Geometry check sheet. Reference: the model listing, model coordinates, mm. Face numbers are marked on the shaded views. A direction names the side the tool comes from. Coordinates: 2 decimals unless noted, no trailing zeros. Order: outer loops, then holes, each group sorted by start corner. A loop starts at its lowest first (then second) coordinate and runs counter-clockwise, first axis right, second up.
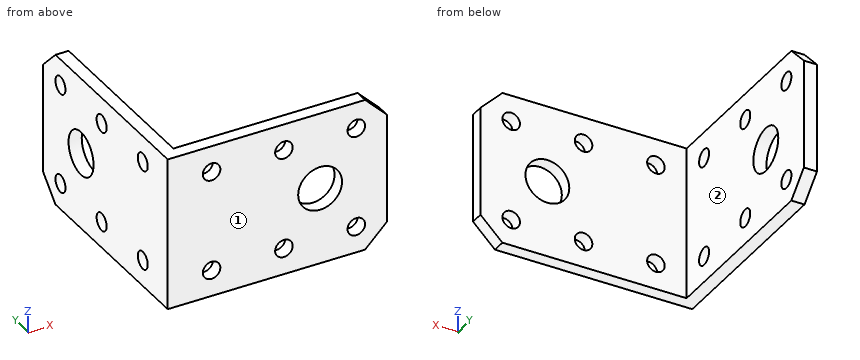
```python
from build123d import *

# Parameters (mm, degrees)
F1_DEPTH = 35
F2_R     = 5
F2_R_2   = 2
F3_DEPTH = 3
F4_R     = 5
F4_R_2   = 2
F5_DEPTH = 3
F6_SIZE  = 5
F7_SIZE  = 5


with BuildPart() as f1:
    # F0 (on Top) → F1 (new body)
    with BuildSketch(Plane.XY):
        Polygon((0, 50), (0, 0), (50, 0), (50, 3), (3, 3), (3, 50), align=None)
    extrude(amount=F1_DEPTH)

    # F2 (on face) → F3 (cut, through all)
    with BuildSketch(Plane(origin=(0, 3, 0), x_dir=(-1, 0, 0), z_dir=(0, 1, 0))):
        with Locations((-34.75, 17.5)):
            Circle(F2_R)
        with Locations((-43, 29)):
            Circle(F2_R_2)
        with Locations((-26.5, 29)):
            Circle(F2_R_2)
        with Locations((-10, 29)):
            Circle(F2_R_2)
        with Locations((-43, 6)):
            Circle(F2_R_2)
        with Locations((-26.5, 6)):
            Circle(F2_R_2)
        with Locations((-10, 6)):
            Circle(F2_R_2)
    extrude(amount=-F3_DEPTH, mode=Mode.SUBTRACT)

    # F4 (on face) → F5 (cut, through all)
    with BuildSketch(Plane.YZ.offset(3)):
        with Locations((34.75, 17.5)):
            Circle(F4_R)
        with Locations((10, 29)):
            Circle(F4_R_2)
        with Locations((26.5, 29)):
            Circle(F4_R_2)
        with Locations((43, 29)):
            Circle(F4_R_2)
        with Locations((10, 6)):
            Circle(F4_R_2)
        with Locations((26.5, 6)):
            Circle(F4_R_2)
        with Locations((43, 6)):
            Circle(F4_R_2)
    extrude(amount=-F5_DEPTH, mode=Mode.SUBTRACT)

    # F6
    f6_edges = [f1.edges().sort_by_distance(p)[0] for p in [
        (50, 1.5, 35),
        (50, 1.5, 0),
    ]]
    chamfer(f6_edges, length=F6_SIZE)

    # F7
    f7_edges = [f1.edges().sort_by_distance(p)[0] for p in [
        (1.5, 50, 35),
        (1.5, 50, 0),
    ]]
    chamfer(f7_edges, length=F7_SIZE)


solid = f1.part
```
Item 1: Sectioned sample at A-A (x = 34.75). Record the cut outline in (y, z), and give its area (3 significant figures).
Item 2: Tool access check on the marked faces 1 and 2. Record the directions out of +Z, -Z, +X, -X, +Y, -Y that give a thin tool (end or side, any length) a straight path to the whole face; none if there is none.
Item 3: Depth check by flat-ended pin: P1, Ø4.5, axis at y = 43, z = 29, coming from the -X side; P2, Ø2.5, axis at x = 43, z = 29, coming from the -Y side; P3, Ø10, axis at x = 17.5, z = 19, coming from the +Y side; P4, Ø10.5, axis at y = 16, z = 19, coming from the +X side. Enter the tip coordinate at first touch or a pass-through.
Item 4: Thickness scan on line 1 along Z through (x, y) = (10, 1.6); line 2 along Z through (x, y) = (34.75, 2.3); line 3 along Y through (x, z) = (19, 18). Record the ranges inside material, lowest first.
Item 5: Sectioned sample at D-D (x = 43). Record the cut outline in (y, z), and give its area (3 significant figures).
Item 6: Sectioned sample at C-C (z = 29). Give the number of separate pieces and of enclosed holes in the cut face, and give its area (3 significant figures).
Geometry check:
1. outline: (0, 0) - (3, 0) - (3, 12.5) - (0, 12.5) - close; (0, 22.5) - (3, 22.5) - (3, 35) - (0, 35) - close
1. area: 75.0 mm2
2. face 1: +Z, -Z, +X, -X, -Y
2. face 2: +Z, -Z, +X, +Y
3. P1: stops at x = 0
3. P2: passes through
3. P3: stops at y = 3
3. P4: stops at x = 3
4. line 1: z = 0 to 4, 8 to 27, 31 to 35
4. line 2: z = 0 to 12.5, 22.5 to 35
4. line 3: y = 0 to 3
5. outline: (0, 0) - (3, 0) - (3, 4) - (0, 4) - close; (0, 8) - (3, 8) - (3, 27) - (0, 27) - close; (0, 31) - (3, 31) - (3, 35) - (0, 35) - close
5. area: 81.0 mm2
6. separate pieces: 7
6. enclosed holes: 0
6. area: 219 mm2
